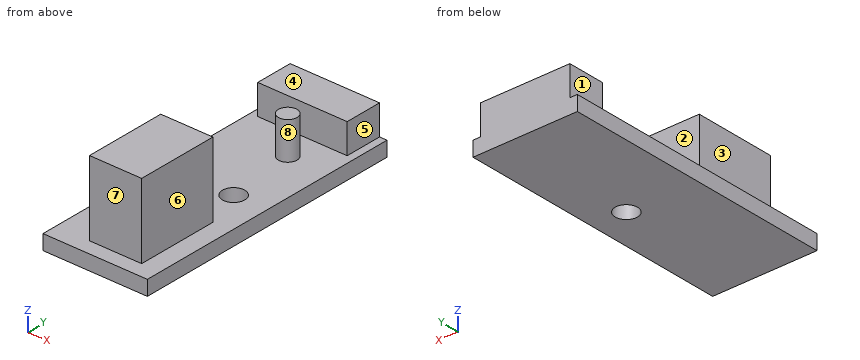
```python
from build123d import *

# Parameters (mm, degrees)
F0_W     = 14
F0_H     = 37
F0_R     = 1.5
F1_DEPTH = 2
F2_W     = 12
F2_H     = 5
F3_DEPTH = 4
F4_R     = 1.25
F5_DEPTH = 5
F6_W     = 7
F6_H     = 11
F7_DEPTH = 10


with BuildPart() as f1:
    # F0 (on Top) → F1 (new body)
    with BuildSketch(Plane.XY):
        with Locations((-2.5, 0)):
            Rectangle(F0_W, F0_H)
        Circle(F0_R, mode=Mode.SUBTRACT)
    extrude(amount=F1_DEPTH)

    # F2 (on face) → F3 (join)
    with BuildSketch(Plane.XY.offset(2)):
        with Locations((-2.5, 16)):
            Rectangle(F2_W, F2_H)
    extrude(amount=F3_DEPTH)

    # F4 (on face) → F5 (join)
    with BuildSketch(Plane.XY.offset(2)):
        with Locations((-1, 9.5)):
            Circle(F4_R)
    extrude(amount=F5_DEPTH)

    # F6 (on face) → F7 (join)
    with BuildSketch(Plane.XY.offset(2)):
        with Locations((-1.5, -11)):
            Rectangle(F6_W, F6_H)
    extrude(amount=F7_DEPTH)


solid = f1.part
```
Input: part model. Units: mm. Frame: model coordinates. Face numbers are marked on the shaded views. A direction names the side the tool comes from. Round coordinates to 2 decimals unless told otherwise and drop trailing zeros. Loops run counter-clockwise (first coordinate to the right, second up) from the corner with the lowest first, then second, coordinate; pieces in that order, holes last.
1) Material intervals for line 1 (Y direction, x = 0, z = 0.5); line 2 (Z direction, x = 3.25, y = -10); line 3 (Y direction, x = -0.25, z = 6.25), sorted ascending.
Ans:
line 1: y = -18.5 to -1.5, 1.5 to 18.5
line 2: z = 0 to 2
line 3: y = -16.5 to -5.5, 8.5 to 10.5
2) Section query A-A on y = 0. Return the cut outline in (x, z).
Ans:
outline: (-9.5, 0) - (-1.5, 0) - (-1.5, 2) - (-9.5, 2) - close; (1.5, 0) - (4.5, 0) - (4.5, 2) - (1.5, 2) - close
3) Pin query (flat end, axial travel): pin 1 (2.5 mm diameter, centred on x = -2.5, y = 16.5, fed in from +Z); pin 2 (1.2 mm diameter, centred on y = 15, z = 4, fed in from -X); pin 3 (1.2 mm diameter, centred on y = 17, z = 5, fed in from +X); pin 4 (1 mm diameter, centred on x = -7, z = 8.5, fed in from +Y). Return the tip coordinate at first contact, or that it passes through.
Ans:
pin 1: stops at z = 6
pin 2: stops at x = -8.5
pin 3: stops at x = 3.5
pin 4: passes through
4) Section query B-B on x = -1. Return the cut outline in (y, z), plus the area to 3 significant figures.
Ans:
outline: (-18.5, 0) - (-1.12, 0) - (-1.12, 2) - (-5.5, 2) - (-5.5, 12) - (-16.5, 12) - (-16.5, 2) - (-18.5, 2) - close; (1.12, 0) - (18.5, 0) - (18.5, 6) - (13.5, 6) - (13.5, 2) - (10.75, 2) - (10.75, 7) - (8.25, 7) - (8.25, 2) - (1.12, 2) - close
area: 212 mm2
5) Pull-direction query (Y, two-part tool) for the marked faces 6, 7 and 8; classes: released by +Y, released by -Y, zero draft, split by the parting line, or undercut.
Ans:
face 6: zero draft
face 7: released by -Y
face 8: undercut
6) Set-up query: the marked faces 1, 2, 3, 4 and 5. Return all of +Z, -Z, +X, -X, +Y, -Y with unobstructed straight access to the full face (end or side cutting, diameter ignored); none if empty.
Ans:
face 1: +Z, -X, +Y, -Y
face 2: +Z, +X, -X
face 3: +Z, -X, -Y
face 4: +Z, +X, -X, +Y
face 5: +Z, +X, +Y, -Y
7) Section query C-C on y = -10. Return the cut outline in (x, z).
Ans:
outline: (-9.5, 0) - (4.5, 0) - (4.5, 2) - (2, 2) - (2, 12) - (-5, 12) - (-5, 2) - (-9.5, 2) - close
8) Section query D-D on z = 8.5. Return the cut outline in (x, y), plus the area to 3 significant figures.
Ans:
outline: (-5, -16.5) - (2, -16.5) - (2, -5.5) - (-5, -5.5) - close
area: 77.0 mm2
